Autodesk Fusion 360 part; units mm, degrees
sketch "Sketch1" plane through (0, 0, 0) normal (1, 0, 0) x (0, 1, 0)
  line L0 (0, 0) -> (200, 0)
  line L1 (200, 0) -> (200, 100)
  line L2 (200, 100) -> (0, 100)
  line L3 (0, 100) -> (0, 0)
extrude "Extrude1" add sketch "Sketch1" along normal blind 50
sketch "Sketch2" plane through (50, 0, 0) normal (1, 0, 0) x (0, 1, 0)
  line L0 (0, 100) -> (0, 0)
  line L1 (0, 0) -> (200, 0)
  line L2 (200, 0) -> (200, 100)
  line L3 (200, 100) -> (0, 100)
shell "Shell1" thickness 5 removed faces 1 at (0, 66.6667, 66.6667)
sketch "Sketch3" plane through (50, 0, 0) normal (1, 0, 0) x (0, 1, 0)
  circle A0 centre (175, 50) radius 5
  line L0 (50, 60) -> (50, 95)
  line L1 (200, 0) -> (200, 100)
  circle A1 centre (130, 20) radius 5
  circle A2 centre (175, 20) radius 5
  circle A3 centre (25, 25) radius 15
  line L2 (195, 95) -> (195, 60)
  circle A4 centre (145, 20) radius 5
  circle A5 centre (145, 35) radius 5
  circle A6 centre (160, 50) radius 5
  circle A7 centre (105, 35) radius 5
  line L3 (0, 0) -> (200, 0)
  circle A8 centre (130, 50) radius 5
  line L4 (200, 100) -> (0, 100)
  line L5 (195, 60) -> (50, 60)
  circle A9 centre (160, 20) radius 5
  circle A10 centre (130, 35) radius 5
  circle A11 centre (105, 50) radius 5
  circle A12 centre (160, 35) radius 5
  circle A13 centre (175, 35) radius 5
  circle A14 centre (145, 50) radius 5
  line L6 (50, 95) -> (195, 95)
  line L7 (0, 100) -> (0, 0)
  circle A15 centre (25, 25) radius 12.5
  point P0 (30, 85)
  point P1 (30, 70)
  point P2 (30, 90)
  point P3 (15, 85)
  point P4 (25, 90)
  point P5 (30, 75)
  point P6 (15, 70)
  point P7 (35, 85)
  point P8 (20, 85)
  point P9 (20, 80)
  point P10 (15, 80)
  point P11 (35, 80)
  point P12 (25, 85)
  point P13 (15, 75)
  point P14 (20, 75)
  point P15 (35, 90)
  point P16 (20, 90)
  point P17 (25, 75)
  point P18 (35, 75)
  point P19 (30, 80)
  point P20 (15, 90)
  point P21 (25, 80)
  point P22 (25, 70)
  point P23 (20, 70)
  point P24 (35, 70)
  dimension "d8" = 10
  dimension "d9" = 10
  dimension "d10" = 10
  dimension "d11" = 30
  dimension "d21" = 25
hole "Hole1" at (50, 35, 90) at (0, 0, 0) at (0, 0, 0) at (0, 0, 0) at (0, 0, 0) at (0, 0, 0) at (0, 0, 0) at (0, 0, 0) at (50, 15, 70) at (0, 0, 0) at (0, 0, 0) at (0, 0, 0) at (50, 25, 85) at (50, 20, 85) at (50, 25, 80) at (50, 25, 75) at (50, 25, 70) at (50, 30, 70) at (50, 30, 75) at (50, 30, 80) at (50, 30, 85) at (50, 35, 85) at (50, 35, 80) at (50, 35, 75) at (50, 35, 70) direction (-1, 0, 0) diameter 3 depth 5 tip angle 180
extrude "Extrude2" add sketch "Sketch3" along normal blind 3 contours L0 L2 L5 L6
extrude "Extrude3" add sketch "Sketch3" along normal blind 3 contours A11
extrude "Extrude4" add sketch "Sketch3" along normal blind 3 contours A0 | A1 | A2 | A4 | A5 | A6 | A7 | A8 | A9 | A10 | A12 | A13 | A14
extrude "Extrude5" add sketch "Sketch3" along normal blind 5 contours A3
extrude "Extrude6" add sketch "Sketch3" along normal blind 3 contours A15
Read the model definition and answer for the solid it produces. Units are mm, in the model's axes. A direction names the side the tool comes from. Round coordinates to 2 decimals unless told otherwise and drop trailing zeros. Order: outer loops, then holes, each group sorted by start corner. A loop starts at its lowest first (then second) coordinate and runs counter-clockwise, first axis right, second up. Notation, with made-up numbers: (72.5, 79) - (101.5, 79) arc R15 cw to (101.5, 87) - close; hole circle Ø10 at (18.25, 28). An arc over 180 degrees is marked (long way). Use one line per item in the form item = value. Start each with the question number.
(1) Flat-ended cylindrical pins translate along their axes: pin 1 Ø11 at (y, z) = (128, 50.5) entering from +X; pin 2 Ø3.5 at (y, z) = (30, 80) entering from +X; pin 3 Ø3.5 at (x, y) = (52, 118) entering from +Z. Find the tip coordinate at first contact, or state that the pin passes through.
(2) The part is cut by section B-B (y = 145). Give the vertices of the cut face in (x, z).
(3) Find the intervals of material crossed by line 1 along Z through (x, y) = (48, 35); line 2 along Y through (x, z) = (46.6, 75); line 3 along Y through (x, z) = (48, 85), in increasing order. Write a range as from..to.
(4) The part is cut by section A-A (x = 33.5). Give the vertices of the cut face in (y, z), then the cut area to 3 significant figures.
(5) For faces 4 (the face through (50, 99, 40)), 5 (the face through (53, 130, 20)), 6 (the face through (22, 195, 49)), determine the directions among +Z, -Z, +X, -X, +Y, -Y from which every point of the face is accessible in a straight line to the end or side of a thin tool.
(6) The part is cut by section C-C (z = 50). Give the vertices of the cut face in (x, y), then the cut area to 3 significant figures.
(7) Determine the mould class of faces 1 (the face through (25, 101, 100)), 2 (the face through (53.986, 15.08, 32.606)), 3 (the face through (53, 175, 35)) for opening direction Z: +Z half, -Z half, draft (parallel to the pull), parting line (faces both ways), or undercut.
(8) The part is cut by section D-D (y = 78.5). Give the vertices of the cut face in (x, z), then the cut area to 4 significant figures.
Checked values:
q1.pin_1 = 53
q1.pin_2 = 50
q1.pin_3 = 95
q2.outline = (0, 0) - (50, 0) - (50, 15) - (53, 15) - (53, 25) - (50, 25) - (50, 30) - (53, 30) - (53, 40) - (50, 40) - (50, 45) - (53, 45) - (53, 55) - (50, 55) - (50, 60) - (53, 60) - (53, 95) - (50, 95) - (50, 100) - (0, 100) - (0, 95) - (45, 95) - (45, 5) - (0, 5) - close
q3.line_1 = 0..68.5, 71.5..73.5, 76.5..78.5, 81.5..83.5, 86.5..88.5, 91.5..100
q3.line_2 = 0..23.5, 26.5..28.5, 31.5..33.5, 36.5..200
q3.line_3 = 0..18.5, 21.5..23.5, 26.5..28.5, 31.5..33.5, 36.5..200
q4.outline = (0, 0) - (200, 0) - (200, 100) - (0, 100) - close; hole (5, 5) - (195, 5) - (195, 95) - (5, 95) - close
q4.area = 2,900 mm^2
q5.face_4 = +X
q5.face_5 = +Z, -Z, +X, +Y
q5.face_6 = -X
q6.outline = (0, 0) - (50, 0) - (50, 100) - (53, 100) - (53, 110) - (50, 110) - (50, 125) - (53, 125) - (53, 135) - (50, 135) - (50, 140) - (53, 140) - (53, 150) - (50, 150) - (50, 155) - (53, 155) - (53, 165) - (50, 165) - (50, 170) - (53, 170) - (53, 180) - (50, 180) - (50, 200) - (0, 200) - (0, 195) - (45, 195) - (45, 5) - (0, 5) - close
q6.area = 1,600 mm^2
q7.face_1 = +Z half
q7.face_2 = undercut
q7.face_3 = draft
q8.outline = (0, 0) - (50, 0) - (50, 60) - (53, 60) - (53, 95) - (50, 95) - (50, 100) - (0, 100) - (0, 95) - (45, 95) - (45, 5) - (0, 5) - close
q8.area = 1,055 mm^2
